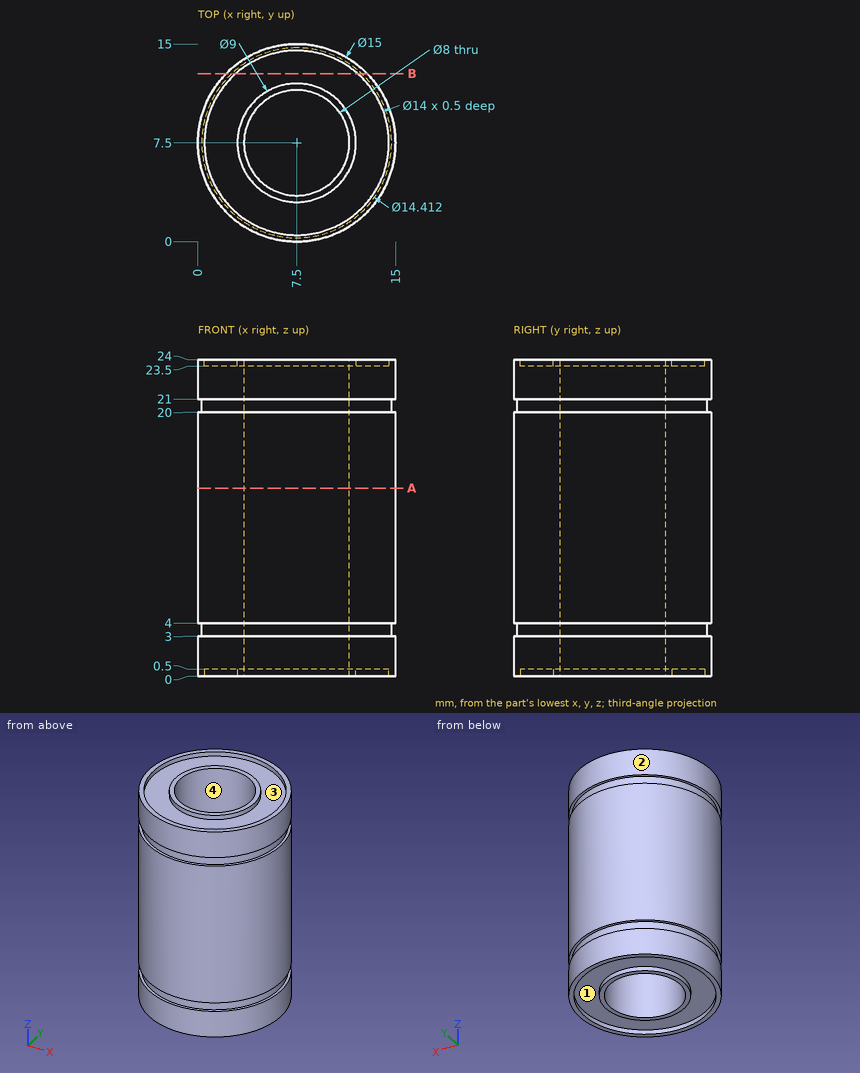
Could you check a few things on this drawing? It's one solid part, dimensions in mm from its lowest x, y, z. A direction names the side the tool comes from. Coordinates: 2 decimals unless noted, no trailing zeros. Loops run counter-clockwise (first coordinate to the right, second up) from the corner with the lowest first, then second, coordinate; pieces in that order, holes last. Notation, with made-up numbers: (38.5, -12) - (44.5, -12) arc R33 ccw to (44.5, 17) - close; hole circle Ø8 at (24, -38). An arc over 180 degrees is marked (long way). Return JSON: item names as keys, results as strings. Group by question number.
Item 1: I need wall thicknesses on line 1 (Y direction, x = 7.5, z = 0.1); line 2 (Z direction, x = 14.25, y = 10.5); line 3 (Z direction, x = 3.5, y = 2.75). Which ranges of each line are inside material? Lowest first, please. Write a range as from..to.
Item 2: If we section it at B-B on y = 12.75: Write out the boundary of the cut face in (x, z).
Item 3: If we section it at A-A on z = 14.25: Write out the boundary of the cut face in (x, y).
Item 4: We'd pull the mould along Y, two halves only. Please class the marked faces 1 and 2: +Y half, -Y half, draft (parallel to the pull), parting line (faces both ways), or undercut.
Item 5: Will these pins go through, and if not, where does the flat tip stop? P1, Ø1, axis at y = 2, z = 13.5, coming from the -X side; P2, Ø5, axis at x = 10, z = 3, coming from the -Y side; P3, Ø2, axis at y = 11.5, z = 6.5, coming from the +X side; P4, Ø8, axis at y = 2, z = 9, coming from the -X side.
Item 6: On a 3-axis mill with a long thin cutter (end or side, diameter ignored), from which of +Z, -Z, +X, -X, +Y, -Y can I reach the whole of each face in a straight line? I mean the marked faces 3 and 4. Say none if no direction works.
Calculated:
{
 "1": {"line 1": "y = 0..0.5, 3..3.5, 11.5..12, 14.5..15", "line 2": "z = 0..3, 4..20, 21..24", "line 3": "z = 0.5..23.5"},
 "2": {"outline": "(2.14, 0) - (2.87, 0) - (2.87, 0.5) - (12.13, 0.5) - (12.13, 0) - (12.86, 0) - (12.86, 3) - (12.44, 3) - (12.44, 4) - (12.86, 4) - (12.86, 20) - (12.44, 20) - (12.44, 21) - (12.86, 21) - (12.86, 24) - (12.13, 24) - (12.13, 23.5) - (2.87, 23.5) - (2.87, 24) - (2.14, 24) - (2.14, 21) - (2.56, 21) - (2.56, 20) - (2.14, 20) - (2.14, 4) - (2.56, 4) - (2.56, 3) - (2.14, 3) - close"},
 "3": {"outline": "circle Ø15 at (7.5, 7.5); hole circle Ø8 at (7.5, 7.5)"},
 "4": {"face 1": "undercut", "face 2": "parting line"},
 "5": {"P1": "stops at x = 1.91", "P2": "stops at y = 0", "P3": "stops at x = 14.37", "P4": "stops at x = 0.15"},
 "6": {"face 3": "+Z", "face 4": "+Z, -Z"}
}
